from build123d import *
from build123d.topology import SkipClean

# Parameters (mm, degrees)
LEFT_ARM_DEPTH                = 12.5
SKETCH2_R                     = 37.5
LEFT_BOSS_DEPTH               = 30
LEFT_HEX_DEPTH                = 262.916017
LEFT_HEX_DEPTH_BACK           = 262.916017
SKETCH3_R                     = 50
CENTRE_BOSS_DEPTH             = 35
SKETCH5_W                     = 25
SKETCH5_H                     = 40
RIGHT_ARM_DEPTH               = 200
SKETCH7_R                     = 50
RIGHT_BOSS_DEPTH              = 30
SKETCH8_R                     = 34
RIGHT_BOSS_HOLE_DEPTH         = 460.541879
SKETCH9_R                     = 40
CENTRE_HOLE_DEPTH             = 461.27572
SKETCH10_R                    = 27.5
CENTRE_BLOB_DEPTH             = 35
CENTRE_BEAM_REACH             = 265.428
SKETCH11_W                    = 50
SKETCH11_H                    = 30
CENTRE_BEAM_DIRECTION_2_REACH = 265.428
SKETCH12_R                    = 20
CUT_EXTRUDE4_DEPTH            = 5
F_1_4_20_TAPPED_HOLE1_D       = 5.1054
CIRPATTERN1_COUNT             = 8
CUT_OUT_DEPTH                 = 10
FILLET1_R                     = 10
FILLET1_OF_MIRROR2_R          = 10


with BuildPart() as part:
    # Sketch1 → LEFT_ARM (new, symmetric)
    with BuildSketch(Plane.XY):
        with BuildLine():
            Line((-2.34375, 37.426686), (196.875, 49.902248))
            ThreePointArc((196.875, 49.902248), (250, 0), (196.875, -49.902248))
            Line((196.875, -49.902248), (-2.34375, -37.426686))
            ThreePointArc((-2.34375, -37.426686), (-37.5, 0), (-2.34375, 37.426686))
        make_face()
    extrude(amount=LEFT_ARM_DEPTH, both=True)

    # Sketch2 → LEFT_Boss (add, symmetric)
    with SkipClean():  # the faces are left unmerged after this step: merging them gives an invalid solid
        with BuildSketch(Plane.XY):
            Circle(SKETCH2_R)
        extrude(amount=LEFT_BOSS_DEPTH, both=True)

    # Sketch4 → LEFT_Hex (cut, two sides: drawn at the far end of the back side and taken through both)
    with SkipClean():  # the faces are left unmerged after this step: merging them gives an invalid solid
        with BuildSketch(Plane.XY.offset(30).offset(-LEFT_HEX_DEPTH_BACK)):
            Polygon((23.094011, 0), (11.547005, 20), (-11.547005, 20), (-23.094011, 0), (-11.547005, -20), (11.547005, -20), align=None)
        extrude(amount=LEFT_HEX_DEPTH + LEFT_HEX_DEPTH_BACK, mode=Mode.SUBTRACT)

    # Sketch3 → CENTRE_Boss (add, symmetric)
    with SkipClean():  # the faces are left unmerged after this step: merging them gives an invalid solid
        with BuildSketch(Plane.XY):
            with Locations((200, 0)):
                Circle(SKETCH3_R)
        extrude(amount=CENTRE_BOSS_DEPTH, both=True)

    # Sketch5 → RIGHT_ARM (add)
    with SkipClean():  # the faces are left unmerged after this step: merging them gives an invalid solid
        with BuildSketch(Plane(origin=(193.969262, -34.202014, 0), x_dir=(0, 0, -1), z_dir=(0.984807753012208, -0.17364817766693072, 0))):
            with Locations((0, 34.729636)):
                Rectangle(SKETCH5_W, SKETCH5_H)
        extrude(amount=RIGHT_ARM_DEPTH)

    # Sketch7 → RIGHT_Boss (add, symmetric)
    with SkipClean():  # the faces are left unmerged after this step: merging them gives an invalid solid
        with BuildSketch(Plane.XY):
            with Locations((396.961551, -34.729636)):
                Circle(SKETCH7_R)
        extrude(amount=RIGHT_BOSS_DEPTH, both=True)

    # Sketch8 → RIGHT_Boss_Hole (cut, through all)
    with SkipClean():  # the faces are left unmerged after this step: merging them gives an invalid solid
        with BuildSketch(Plane.XY.offset(30)):
            with Locations((396.961551, -34.729636)):
                Circle(SKETCH8_R)
        extrude(amount=-RIGHT_BOSS_HOLE_DEPTH, mode=Mode.SUBTRACT)

    # Sketch9 → CENTRE_Hole (cut, through all)
    with SkipClean():  # the faces are left unmerged after this step: merging them gives an invalid solid
        with BuildSketch(Plane.XY.offset(35)):
            with Locations((200, 0)):
                Circle(SKETCH9_R)
        extrude(amount=-CENTRE_HOLE_DEPTH, mode=Mode.SUBTRACT)

    # Sketch10 → CENTRE_Blob (add, symmetric)
    with SkipClean():  # the faces are left unmerged after this step: merging them gives an invalid solid
        with BuildSketch(Plane.XY):
            with Locations((224.620194, -4.341204)):
                Circle(SKETCH10_R)
        extrude(amount=CENTRE_BLOB_DEPTH, both=True)

    # Sketch11 → CENTRE_Beam (add, up to next)
    with BuildSketch(Plane(origin=(200, 0, 0), x_dir=(0, 0, -1), z_dir=(1, 0, 0)), mode=Mode.PRIVATE) as centre_beam_sk1:
        Rectangle(SKETCH11_W, SKETCH11_H)
    centre_beam_tool1 = extrude(centre_beam_sk1.sketch, amount=CENTRE_BEAM_REACH, mode=Mode.PRIVATE) - part.part
    add(centre_beam_tool1.solids().sort_by_distance((200, 0, 0))[0])

    # Sketch11 → CENTRE_Beam direction 2 (add, up to next)
    with BuildSketch(Plane(origin=(200, 0, 0), x_dir=(0, 0, -1), z_dir=(1, 0, 0)), mode=Mode.PRIVATE) as centre_beam_direction_2_sk1:
        Rectangle(SKETCH11_W, SKETCH11_H)
    centre_beam_direction_2_tool1 = extrude(centre_beam_direction_2_sk1.sketch, amount=-CENTRE_BEAM_DIRECTION_2_REACH, mode=Mode.PRIVATE) - part.part
    add(centre_beam_direction_2_tool1.solids().sort_by_distance((200, 0, 0))[0])

    # Sketch12 → Cut-Extrude4 (cut)
    with SkipClean():  # the faces are left unmerged after this step: merging them gives an invalid solid
        with BuildSketch(Plane.XY.offset(35)):
            with Locations((224.620194, -4.341204)):
                Circle(SKETCH12_R)
        cut_extrude4 = extrude(amount=-CUT_EXTRUDE4_DEPTH, mode=Mode.SUBTRACT)

    # 1/4-20 Tapped Hole1 (through all)
    with Locations(Plane.XY.offset(30)):
        with Locations((209.848078, -1.736482)):
            f_1_4_20_tapped_hole1 = Hole(F_1_4_20_TAPPED_HOLE1_D / 2)

    # CirPattern1: 1/4-20 Tapped Hole1 ×8 about axis
    with SkipClean():  # the faces are left unmerged after this step: merging them gives an invalid solid
        cirpattern1_axis = Axis((224.620194, -4.341204, 0), (0, 0, 1))
        for i in range(1, CIRPATTERN1_COUNT):
            add(f_1_4_20_tapped_hole1.rotate(cirpattern1_axis, i * 360 / CIRPATTERN1_COUNT), mode=Mode.SUBTRACT)

    # Mirror1: Cut-Extrude4 across plane
    with SkipClean():  # the faces are left unmerged after this step: merging them gives an invalid solid
        add(cut_extrude4.mirror(Plane.XY), mode=Mode.SUBTRACT)

    # Sketch15 → Cut_OUT (cut)
    with SkipClean():  # the faces are left unmerged after this step: merging them gives an invalid solid
        with BuildSketch(Plane.XY.offset(12.5)):
            with BuildLine():
                Line((152.866072, 37.126714), (36.935365, 29.866851))
                ThreePointArc((36.935365, 29.866851), (47.5, 0), (36.935365, -29.866851))
                Line((36.935365, -29.866851), (152.866072, -37.126714))
                ThreePointArc((152.866072, -37.126714), (140, 0), (152.866072, 37.126714))
            make_face()
        cut_out = extrude(amount=-CUT_OUT_DEPTH, mode=Mode.SUBTRACT)

    # Fillet1
    fillet1_edges = [part.edges().sort_by_distance(p)[0] for p in [
        (36.935365, -29.866851, 7.5),
        (36.935365, 29.866851, 7.5),
        (152.866072, 37.126714, 7.5),
        (152.866072, -37.126714, 7.5),
    ]]
    fillet(fillet1_edges, radius=FILLET1_R)

    # Mirror2: Cut_OUT across plane
    with SkipClean():  # the faces are left unmerged after this step: merging them gives an invalid solid
        add(cut_out.mirror(Plane.XY), mode=Mode.SUBTRACT)

    # Fillet1 of Mirror2
    fillet1_of_mirror2_edges = [part.edges().sort_by_distance(p)[0] for p in [
        (36.935365, -29.866851, -7.5),
        (36.935365, 29.866851, -7.5),
        (152.866072, 37.126714, -7.5),
        (152.866072, -37.126714, -7.5),
    ]]
    fillet(fillet1_of_mirror2_edges, radius=FILLET1_OF_MIRROR2_R)


solid = part.part
Could you check a few things on this model? Use its own coordinates, in mm. A direction names the side the tool comes from. Give positions to 0.01 mm unless a question says otherwise; leave off trailing zeros. Order: outer loops, then holes, each group sorted by start corner. A loop starts at its lowest first (then second) coordinate and runs counter-clockwise, first axis right, second up.
1. I need wall thicknesses on L1, parallel to X at y = -8.5, z = 11.5 (3 decimals); L2, parallel to X at y = -21, z = -31; L3, parallel to X at y = -10, z = 28. Which ranges of each line are inside material? Lowest first, please.
Answers below:
L1: x = -36.524 to -18.187, 18.187 to 46.733, 140.605 to 237.367, 241.417 to 375.328, 418.595 to 439.529
L2: x = 154.62 to 165.96, 202.74 to 213.55, 235.69 to 246.5
L3: x = -36.14 to -17.32, 17.32 to 36.14, 151.01 to 161.27, 197.71 to 251.53, 353.51 to 373.63, 420.29 to 440.42
2. For pin 1 (9 mm diameter, centred on x = 175, y = 1, fed in from -Z); pin 2 (12 mm diameter, centred on x = 129, z = 12, fed in from +Y); pin 3 (12 mm diameter, centred on x = 216, y = 4.5, fed in from -Z), each with a flat end and sliding along its axis, tell me the tip position at first contact or that it passes through.
Answers below:
pin 1: stops at z = -25
pin 2: stops at y = 46.03
pin 3: stops at z = -30
3. Suppose I cut it at A-A (z = 18). State how many separate pieces and enclosed holes the cut face has, plus the area to 3 significant figures.
Answers below:
separate pieces: 3
enclosed holes: 12
area: 12,900 mm2
4. Suppose I cut it at B-B (x = 382.5). Write out the boundary of the cut face in (y, z), plus the area to 3 significant figures.
Answers below:
outline: (-82.59, -30) - (-65.5, -30) - (-65.5, 30) - (-82.59, 30) - close; (-3.96, -30) - (13.13, -30) - (13.13, 30) - (-3.96, 30) - close
area: 2,050 mm2
5. Thinking about a two-plate mould opening in X: for faces 1 (the cylindrical face through (251.66, -9.35, 23.91)), 2 (the flat face through (430, -45, 30)), which applies, +X half, -X half, draft (parallel to the pull), parting line (faces both ways), or undercut?
Answers below:
face 1: undercut
face 2: draft
6. Suppose I cut it at C-C (x = 94.5). Write out the boundary of the cut face in (y, z), plus the area to 3 significant figures.
Answers below:
outline: (-43.49, -12.5) - (-33.47, -12.5) - (-33.47, -2.5) - (33.47, -2.5) - (33.47, -12.5) - (43.49, -12.5) - (43.49, 12.5) - (33.47, 12.5) - (33.47, 2.5) - (-33.47, 2.5) - (-33.47, 12.5) - (-43.49, 12.5) - close
area: 836 mm2
7. Suppose I cut it at D-D (y = -76). Write out the boundary of the cut face in (x, z).
Answers below:
outline: (368.73, -30) - (425.19, -30) - (425.19, 30) - (368.73, 30) - close
8. Which directions (+Z, -Z, +X, -X, +Y, -Y) give clear straight access to the entire face, cutting with the end or side of a thin tool? Please do faces 3 (the flat face through (16, -16, -30)), 4 (the flat face through (17.4, 9.86, -0.42)), 5 (the flat face through (16, -16, 30)).
Answers below:
face 3: -Z, -X, +Y, -Y
face 4: +Z, -Z
face 5: +Z, -X, +Y, -Y
